```python
from build123d import *

# Parameters (mm, degrees)
SALIENTE_EXTRUIR1_DEPTH       = 19.05
TALADRO_DE_MARGEN_PARA_1_41_D = 6.7564


with BuildPart() as part:
    # Croquis1 → Saliente-Extruir1 (new, symmetric)
    with BuildSketch(Plane.XY):
        Polygon((0, 0), (-90, 0), (-327.587878479, 237.587878479), (-329.002092041, 236.173664916), (-90.828427125, -2), (0, -2), align=None)
    extrude(amount=SALIENTE_EXTRUIR1_DEPTH, both=True)

    # Taladro de margen para 1/41 (through all)
    with Locations(Plane(origin=(-70, 0, 0), x_dir=(1, 0, 0), z_dir=(0, 1, 0))):
        with Locations((0, 0), (40, 0)):
            Hole(TALADRO_DE_MARGEN_PARA_1_41_D / 2)


solid = part.part
```
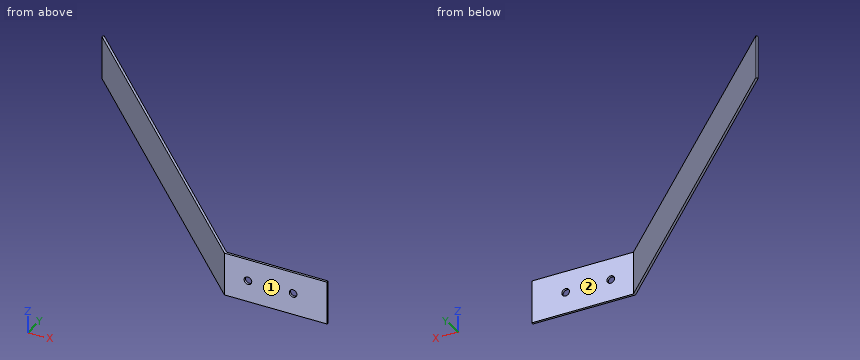
Work out the finished part from the listing and answer in its coordinate system (mm). Face numbers are marked on the shaded views. A direction names the side the tool comes from. Give positions to 0.01 mm unless a question says otherwise; leave off trailing zeros. Order: outer loops, then holes, each group sorted by start corner. A loop starts at its lowest first (then second) coordinate and runs counter-clockwise, first axis right, second up.
1. Section D-D, the plane x = -250 is taken. Determine the outline of the cut face in (y, z), and give its area (3 significant figures).
Result sheet:
outline: (157.17, -19.05) - (160, -19.05) - (160, 19.05) - (157.17, 19.05) - close
area: 108 mm2
2. Section A-A, the plane x = -70 is taken. Determine the outline of the cut face in (y, z).
Result sheet:
outline: (-2, -19.05) - (0, -19.05) - (0, -3.38) - (-2, -3.38) - close; (-2, 3.38) - (0, 3.38) - (0, 19.05) - (-2, 19.05) - close
3. For the marked faces 1 and 2, determine the directions among +Z, -Z, +X, -X, +Y, -Y from which every point of the face is accessible in a straight line to the end or side of a thin tool.
Result sheet:
face 1: +Z, -Z, +X, -X, -Y
face 2: +Z, -Z, +X, +Y
4. Straight lines are drawn through the part: L1, parallel to Z at x = -70, y = -1.1; L2, parallel to Y at x = -59, z = 17; L3, parallel to X at y = 100, z = -0.5. For each, find the intervals that lie inside material, in ascending order.
Result sheet:
L1: z = -19.05 to -3.38, 3.38 to 19.05
L2: y = -2 to 0
L3: x = -192.83 to -190
5. Section C-C, the plane y = 200 is taken. Determine the outline of the cut face in (x, z), and give its area (3 significant figures).
Result sheet:
outline: (-292.83, -19.05) - (-290, -19.05) - (-290, 19.05) - (-292.83, 19.05) - close
area: 108 mm2
6. Section B-B, the plane z = 0 is taken. Determine the outline of the cut face in (x, y), and give its area (3 significant figures).
Result sheet:
outline: (-329, 236.17) - (-90.83, -2) - (-73.38, -2) - (-73.38, 0) - (-90, 0) - (-327.59, 237.59) - close; (-66.62, -2) - (-33.38, -2) - (-33.38, 0) - (-66.62, 0) - close; (-26.62, -2) - (0, -2) - (0, 0) - (-26.62, 0) - close
area: 827 mm2
7. Each of these flat-tipped pins is pushed along its axis until it touches: P1, Ø4, axis at y = 77, z = -2.5, coming from the +X side; P2, Ø2, axis at y = 81, z = -5.5, coming from the +X side; P3, Ø8, axis at x = -70, z = 0, coming from the -Y side; P4, Ø10, axis at x = -84, z = 8.5, coming from the +Y side. Where does it stop, or does it pass through?
Result sheet:
P1: stops at x = -165
P2: stops at x = -170
P3: stops at y = -2
P4: stops at y = 0
